The model under review builds one solid part; all positions refer to its coordinate system, in mm. Coordinates: 2 decimals unless noted, no trailing zeros. Loops run counter-clockwise (first coordinate to the right, second up) from the corner with the lowest first, then second, coordinate; pieces in that order, holes last. Notation, with made-up numbers: (-28, -3) - (0, -3) arc R26 ccw to (0, 35) - close; hole circle Ø10 at (10.25, 8). An arc over 180 degrees is marked (long way). Answer in a Markdown table with one row per item. Add a question column.
(1) For P1, Ø3, axis at x = 82, z = 2.5, coming from the -Y side; P2, Ø3, axis at x = 137.4, y = 137.4, coming from the +Z side; P3, Ø2.5, axis at x = 135.5, y = 109, coming from the +Z side; P4, Ø1, axis at x = -102.5, z = 3, coming from the +Y side, all flat-tipped, find the tip position at first contact; note any pin that passes through.
(2) For line 1 along Y through (x, z) = (137.4, 4.95); line 2 along Y through (x, z) = (-137.5, 1.75); line 3 along X through (y, z) = (107.5, 5), list the stretches that pass through material, from the lowest coordinate up.
(3) We need section C-C on z = 4.75. Give the number of separate pieces and of enclosed holes in the cut face, plus the area to 3 significant figures.
(4) We need section B-B on y = 36. Write out the cut boundary in (x, z), plus the area to 3 significant figures.
(5) We need section A-A on x = -98. Write out the cut boundary in (y, z), plus the area to 3 significant figures.
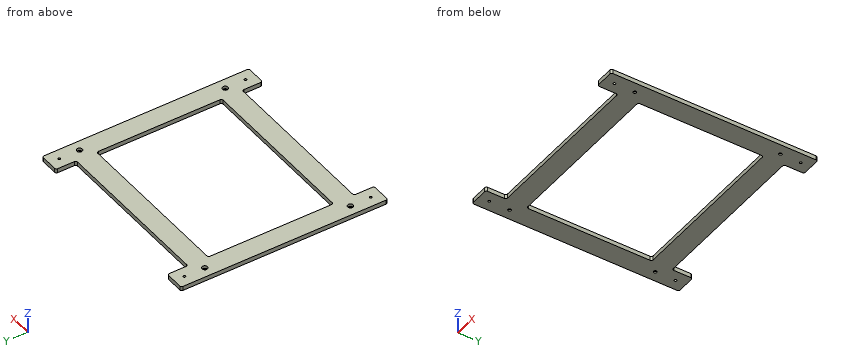
from build123d import *

# Parameters (mm, degrees)
BOSS_EXTRUDE1_DEPTH            = 6.35
CBORE_FOR_M4_SHCS1_D           = 4.5
CBORE_FOR_M4_SHCS1_CBORE_D     = 8
CBORE_FOR_M4_SHCS1_CBORE_DEPTH = 4
M3_CLEARANCE_HOLE2_D           = 3.4


with BuildPart() as part:
    # Sketch7 → Boss-Extrude1 (new body)
    with BuildSketch(Plane.XY):
        with BuildLine():
            Line((-119.9, -122.4), (119.9, -122.4))
            ThreePointArc((119.9, -122.4), (121.667766953, -123.132233047), (122.4, -124.9))
            Line((122.4, -124.9), (122.4, -149.9))
            ThreePointArc((122.4, -149.9), (123.132233047, -151.667766953), (124.9, -152.4))
            Line((124.9, -152.4), (149.9, -152.4))
            ThreePointArc((149.9, -152.4), (151.667766953, -151.667766953), (152.4, -149.9))
            Line((152.4, -149.9), (152.4, -102.186961883))
            Line((152.4, -102.186961883), (152.4, 120.74319893))
            Line((152.4, 120.74319893), (152.4, 149.9))
            ThreePointArc((152.4, 149.9), (151.667766953, 151.667766953), (149.9, 152.4))
            Line((149.9, 152.4), (124.9, 152.4))
            ThreePointArc((124.9, 152.4), (123.132233047, 151.667766953), (122.4, 149.9))
            Line((122.4, 149.9), (122.4, 124.9))
            ThreePointArc((122.4, 124.9), (121.667766953, 123.132233047), (119.9, 122.4))
            Line((119.9, 122.4), (-119.9, 122.4))
            ThreePointArc((-119.9, 122.4), (-121.667766953, 123.132233047), (-122.4, 124.9))
            Line((-122.4, 124.9), (-122.4, 149.9))
            ThreePointArc((-122.4, 149.9), (-123.132233047, 151.667766953), (-124.9, 152.4))
            Line((-124.9, 152.4), (-149.9, 152.4))
            ThreePointArc((-149.9, 152.4), (-151.667766953, 151.667766953), (-152.4, 149.9))
            Line((-152.4, 149.9), (-152.4, 102.186961883))
            Line((-152.4, 102.186961883), (-152.4, -120.74319893))
            Line((-152.4, -120.74319893), (-152.4, -149.9))
            ThreePointArc((-152.4, -149.9), (-151.667766953, -151.667766953), (-149.9, -152.4))
            Line((-149.9, -152.4), (-124.9, -152.4))
            ThreePointArc((-124.9, -152.4), (-123.132233047, -151.667766953), (-122.4, -149.9))
            Line((-122.4, -149.9), (-122.4, -124.9))
            ThreePointArc((-122.4, -124.9), (-121.667766953, -123.132233047), (-119.9, -122.4))
        make_face()
        with BuildLine():
            Line((-119.9, -92.4), (119.9, -92.4))
            ThreePointArc((119.9, -92.4), (121.667766953, -91.667766953), (122.4, -89.9))
            Line((122.4, -89.9), (122.4, 89.9))
            ThreePointArc((122.4, 89.9), (121.667766953, 91.667766953), (119.9, 92.4))
            Line((119.9, 92.4), (-119.9, 92.4))
            ThreePointArc((-119.9, 92.4), (-121.667766953, 91.667766953), (-122.4, 89.9))
            Line((-122.4, 89.9), (-122.4, -89.9))
            ThreePointArc((-122.4, -89.9), (-121.667766953, -91.667766953), (-119.9, -92.4))
        make_face(mode=Mode.SUBTRACT)
    extrude(amount=BOSS_EXTRUDE1_DEPTH)

    # CBORE for M4 SHCS1 (through all)
    with Locations(Plane.XY.offset(6.35)):
        with Locations((-137.4, 107.4), (-137.4, -107.4), (137.4, -107.4), (137.4, 107.4)):
            CounterBoreHole(CBORE_FOR_M4_SHCS1_D / 2, CBORE_FOR_M4_SHCS1_CBORE_D / 2, CBORE_FOR_M4_SHCS1_CBORE_DEPTH)

    # M3 Clearance Hole2 (through all)
    with Locations(Plane.XY.offset(6.35)):
        with Locations((-137.4, 137.4), (137.4, 137.4), (137.4, -137.4), (-137.4, -137.4)):
            Hole(M3_CLEARANCE_HOLE2_D / 2)


solid = part.part
Outcome:
| question | item | result |
|---|---|---|
| 1 | P1 | y = -122.4 |
| 1 | P2 | through |
| 1 | P3 | z = 2.35 |
| 1 | P4 | y = 122.4 |
| 2 | line 1 | -152.4 to -139.1, -135.7 to -111.4, -103.4 to 103.4, 111.4 to 135.7, 139.1 to 152.4 |
| 2 | line 2 | -152.4 to -139.1, -135.7 to -109.65, -105.15 to 105.15, 109.65 to 135.7, 139.1 to 152.4 |
| 2 | line 3 | -152.4 to -141.4, -133.4 to 133.4, 141.4 to 152.4 |
| 3 | separate pieces | 1 |
| 3 | enclosed holes | 9 |
| 3 | area | 32,700 mm² |
| 4 | outline | (-152.4, 0) - (-122.4, 0) - (-122.4, 6.35) - (-152.4, 6.35) - close; (122.4, 0) - (152.4, 0) - (152.4, 6.35) - (122.4, 6.35) - close |
| 4 | area | 381 mm² |
| 5 | outline | (-122.4, 0) - (-92.4, 0) - (-92.4, 6.35) - (-122.4, 6.35) - close; (92.4, 0) - (122.4, 0) - (122.4, 6.35) - (92.4, 6.35) - close |
| 5 | area | 381 mm² |
